```python
from build123d import *

# Parameters (mm, degrees)
F_10_24_TAPPED_HOLE1_D     = 3.7973
CHAMFER1_SIZE              = 0.762
SKETCH5_R                  = 7.9375
CUT_EXTRUDE2_DEPTH         = 25.7077
F_6_32_TAPPED_HOLE2_REACH  = 85.841
F_6_32_TAPPED_HOLE2_BORE_R = 1.35255
SKETCH12_R                 = 12.7
CUT_EXTRUDE3_DEPTH         = 9.525
CUT_EXTRUDE4_DEPTH         = 8.39875
F_6_32_TAPPED_HOLE1_D      = 2.7051
F_6_32_TAPPED_HOLE1_DEPTH  = 15
F_6_32_TAPPED_HOLE1_TIP    = 0.81269403
SKETCH18_R                 = 3.475
CUT_EXTRUDE6_DEPTH         = 1.778
F_10_CLEARANCE_HOLE1_D     = 4.9784
CIRPATTERN1_COUNT          = 6
CHAMFER2_SIZE              = 3
CHAMFER2_SIZE2             = 5.196152423
SKETCH23_R                 = 40.8305
SKETCH23_R_2               = 31.3055
CUT_EXTRUDE7_DEPTH         = 4.7625
FILLET1_R                  = 2.38125
FILLET2_R                  = 4.7625


with BuildPart() as part:
    # Sketch1 → Revolve1 (revolve)
    with BuildSketch(Plane.XY, mode=Mode.PRIVATE) as revolve1_sk:
        Polygon((0, 0), (11.1125, 0), (11.1125, 18.4277), (47.625, 18.4277), (47.625, 20.80895), (42.8625, 20.80895), (42.8625, 29.2077), (47.625, 29.2077), (47.625, 36.2077), (0, 36.2077), align=None)
    revolve(revolve1_sk.sketch.rotate(Axis((0, 36.2077, 0), (0, -1, 0)), 90), axis=Axis((0, 36.2077, 0), (0, -1, 0)))

    # #10-24 Tapped Hole1 (through all)
    with Locations(Plane(origin=(0, 36.2077, 0), x_dir=(1, 0, 0), z_dir=(0, 1, 0))):
        with Locations((0, 0)):
            Hole(F_10_24_TAPPED_HOLE1_D / 2)

    # Chamfer1
    chamfer1_edges = [part.edges().sort_by_distance(p)[0] for p in [
        (0, 29.2077, -47.625),
        (0, 20.80895, -47.625),
    ]]
    chamfer(chamfer1_edges, length=CHAMFER1_SIZE)

    # Sketch5 → Cut-Extrude2 (cut)
    with BuildSketch(Plane(origin=(0, 36.2077, 0), x_dir=(1, 0, 0), z_dir=(0, 1, 0))):
        with Locations(Location((0, 0, 0), (0, 0, 270))):
            Circle(SKETCH5_R)
    extrude(amount=-CUT_EXTRUDE2_DEPTH, mode=Mode.SUBTRACT)

    # #6-32 Tapped Hole2 bore → #6-32 Tapped Hole2 (cut, up to next)
    with BuildSketch(Plane(origin=(0, 0, -11.1125), x_dir=(-1, 0, 0), z_dir=(0, 0, -1)), mode=Mode.PRIVATE) as f_6_32_tapped_hole2_sk1:
        with Locations((0, 8.2677)):
            Circle(F_6_32_TAPPED_HOLE2_BORE_R)
    f_6_32_tapped_hole2_tool1 = extrude(f_6_32_tapped_hole2_sk1.sketch, amount=-F_6_32_TAPPED_HOLE2_REACH, mode=Mode.PRIVATE) & part.part
    add(f_6_32_tapped_hole2_tool1.solids().sort_by_distance((0, 8.2677, -11.1125))[0], mode=Mode.SUBTRACT)

    # Sketch12 → Cut-Extrude3 (cut)
    with BuildSketch(Plane(origin=(0, 36.2077, 0), x_dir=(1, 0, 0), z_dir=(0, 1, 0))):
        with Locations(Location((0, 0, 0), (0, 0, 270))):
            Circle(SKETCH12_R)
    extrude(amount=-CUT_EXTRUDE3_DEPTH, mode=Mode.SUBTRACT)

    # Sketch13 → Cut-Extrude4 (cut)
    with BuildSketch(Plane.XZ.offset(-29.2077)):
        with BuildLine():
            Line((36.5125, 0), (36.5125, -22.450640303))
            ThreePointArc((36.5125, -22.450640303), (41.244459855, -11.6656949), (42.8625, 0))
            Line((42.8625, 0), (36.5125, 0))
        make_face()
    extrude(amount=CUT_EXTRUDE4_DEPTH, mode=Mode.SUBTRACT)

    # #6-32 Tapped Hole1
    with Locations(Plane(origin=(36.5125, 0, 0), x_dir=(0, 0, -1), z_dir=(1, 0, 0))):
        with Locations((3.5, 25.008325)):
            Hole(F_6_32_TAPPED_HOLE1_D / 2, depth=F_6_32_TAPPED_HOLE1_DEPTH)
            with Locations((0, 0, -(F_6_32_TAPPED_HOLE1_DEPTH + F_6_32_TAPPED_HOLE1_TIP / 2))):  # 118° drill point
                Cone(0, F_6_32_TAPPED_HOLE1_D / 2, F_6_32_TAPPED_HOLE1_TIP, mode=Mode.SUBTRACT)

    # Sketch18 → Cut-Extrude6 (cut)
    with BuildSketch(Plane.XZ):
        with Locations(Location((0, 0, 0), (0, 0, 270))):
            Circle(SKETCH18_R)
    extrude(amount=-CUT_EXTRUDE6_DEPTH, mode=Mode.SUBTRACT)

    # #10 Clearance Hole1 (through all)
    with Locations(Plane(origin=(0, 18.4277, 0), x_dir=(-1, 0, 0), z_dir=(0, -1, 0))):
        with Locations((0, -36.2458)):
            f_10_clearance_hole1 = Hole(F_10_CLEARANCE_HOLE1_D / 2)

    # CirPattern1: #10 Clearance Hole1 ×6 about axis
    cirpattern1_axis = Axis((0, 0, 0), (0, 1, 0))
    for i in range(1, CIRPATTERN1_COUNT):
        add(f_10_clearance_hole1.rotate(cirpattern1_axis, i * 360 / CIRPATTERN1_COUNT), mode=Mode.SUBTRACT)

    # Chamfer2
    chamfer2_edges = [part.edges().sort_by_distance(p)[0] for p in [
        (0, 36.2077, -47.625),
    ]]
    chamfer2_side = [part.faces().sort_by_distance(p)[0] for p in [
        (0, 33.0887, -47.625),
    ]]
    chamfer(chamfer2_edges, length=CHAMFER2_SIZE, length2=CHAMFER2_SIZE2, reference=chamfer2_side[0])

    # Sketch23 → Cut-Extrude7 (cut)
    with BuildSketch(Plane(origin=(0, 36.2077, 0), x_dir=(1, 0, 0), z_dir=(0, 1, 0))):
        with Locations(Location((0, 0, 0), (0, 0, 270))):
            Circle(SKETCH23_R)
        with Locations(Location((0, 0, 0), (0, 0, 270))):
            Circle(SKETCH23_R_2, mode=Mode.SUBTRACT)
    extrude(amount=-CUT_EXTRUDE7_DEPTH, mode=Mode.SUBTRACT)

    # Fillet1
    fillet1_edges = [part.edges().sort_by_distance(p)[0] for p in [
        (0, 31.4452, -31.3055),
        (0, 31.4452, -40.8305),
    ]]
    fillet(fillet1_edges, radius=FILLET1_R)

    # Fillet2
    fillet2_edges = [part.edges().sort_by_distance(p)[0] for p in [
        (36.5125, 25.008325, -22.450640303),
    ]]
    fillet(fillet2_edges, radius=FILLET2_R)


solid = part.part
```
Read the model definition and answer for the solid it produces. Units are mm, in the model's axes. A direction names the side the tool comes from. Round coordinates to 2 decimals unless told otherwise and drop trailing zeros. Write each loop counter-clockwise with the first axis right and the second up, starting at its lowest first coordinate (ties: lowest second). Pieces come first, ordered by that corner, then holes. Notation, with made-up numbers: (74.5, -14) -> (112.5, -14) arc R18 ccw to (112.5, -9) -> close; hole circle Ø11 at (-6.5, 13). An arc over 180 degrees is marked (long way). Answer in a Markdown table with one row per item. Add a question column.
1) Consider line 1 (Y direction, x = 27.5, z = -3.5); line 2 (Z direction, x = 21.5, y = 32.5); line 3 (Y direction, x = -30.5, z = -14.5). Determine where each line is inside the solid, lowest interval first.
2) Find section A-A, the plane y = 12.5. Determine the outline of the cut face in (x, z) (1 decimal).
3) Determine the mould class of faces 1 (the face through (-3.34, 9.34, 10.6)), 2 (the face through (-11.3, 18.428, 0.7)), 3 (the face through (28.9, 25, -18.2)), 4 (the face through (-7.75, 18.7, -1.72)) for opening direction Z: pulls with the +Z half, pulls with the -Z half, needs draft (parallel to the pull), parting line crosses it, or undercut.
4) Which of the six approach directions +Z, -Z, +X, -X, +Y, -Y give full straight-line access (tool end or side, diameter ignored) to faces 5 (the face through (21, 25, -4)), 6 (the face through (38, 29.208, -3)), 7 (the face through (-2, 10.5, 2))?
5) Given P1, Ø5.5, axis at x = -31.39, z = 18.12, coming from the +Y side; P2, Ø4.5, axis at x = 31.39, z = -18.12, coming from the +Y side; P3, Ø6.5, axis at x = -31.39, z = -18.12, coming from the +Y side; P4, Ø4, axis at x = 0, z = 0, coming from the +Y side, each flat-ended and moving along its own axis, determine where each tip first touches the part or whether it passes through.
Findings below:
| question | item | result |
|---|---|---|
| 1 | line 1 | 18.43 to 23.66, 26.36 to 36.21 |
| 1 | line 2 | -42.5 to -34.24, -23.31 to 23.31, 34.24 to 42.5 |
| 1 | line 3 | 18.43 to 31.45 |
| 2 | outline | circle Ø22.2 at (0, 0); hole circle Ø15.9 at (0, 0) |
| 3 | face 1 | parting line crosses it |
| 3 | face 2 | needs draft |
| 3 | face 3 | undercut |
| 3 | face 4 | undercut |
| 4 | face 5 | +X |
| 4 | face 6 | none |
| 4 | face 7 | +Y |
| 5 | P1 | y = 31.49 |
| 5 | P2 | through |
| 5 | P3 | y = 31.67 |
| 5 | P4 | y = 10.5 |
